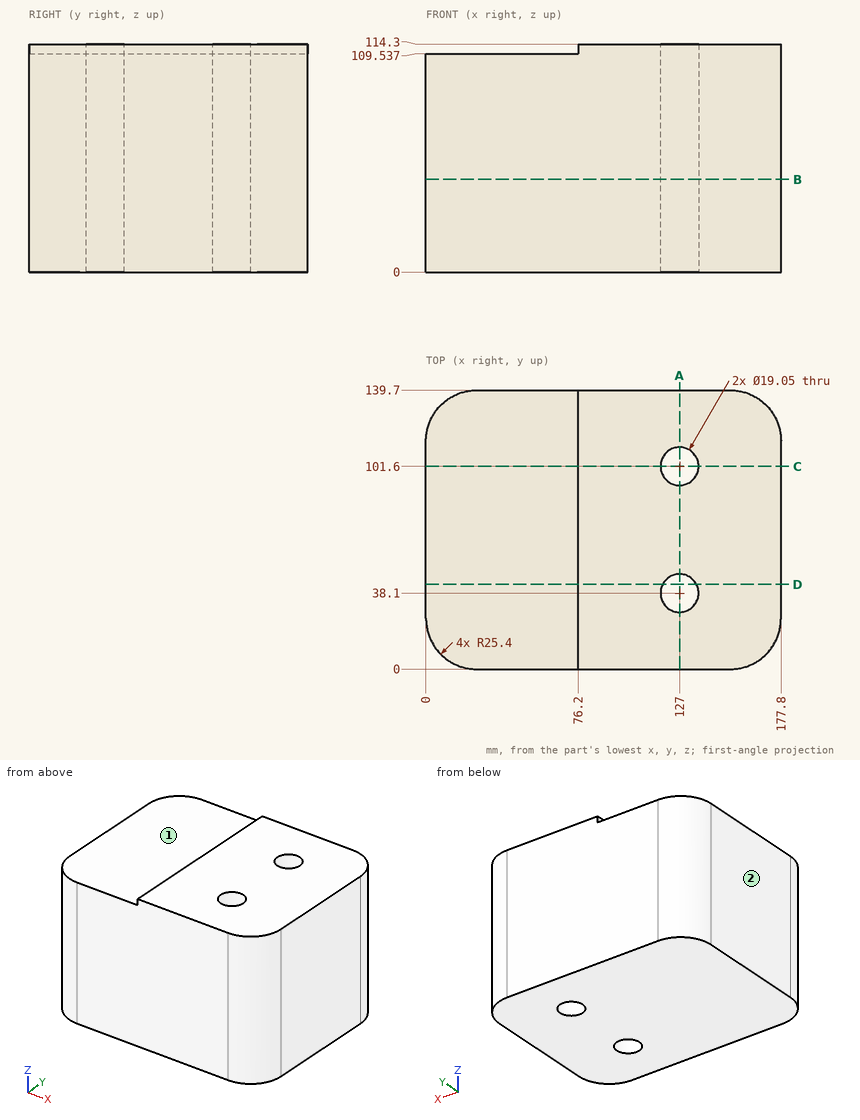
Here's the drawing with two shaded views (mm, measured from the low corner). I have some questions. A direction names the side the tool comes from. Coordinates: 2 decimals unless noted, no trailing zeros. Write each loop counter-clockwise with the first axis right and the second up, starting at its lowest first coordinate (ties: lowest second). Pieces come first, ordered by that corner, then holes.
Item 1: I want a section at C-C on y = 101.6. Write out the boundary of the cut face in (x, z) (1 decimal), and give its area (3 significant figures).
Item 2: Will these pins go through, and if not, where does the flat tip stop? pin 1 (23 mm diameter, centred on x = 25, y = 65.5, fed in from +Z); pin 2 (1 mm diameter, centred on y = 123, z = 100, fed in from -X); pin 3 (2.5 mm diameter, centred on y = 68.5, z = 111.5, fed in from -X).
Item 3: I want a section at A-A on x = 127. Write out the boundary of the cut face in (y, z) (1 decimal).
Item 4: On a 3-axis mill with a long thin cutter (end or side, diameter ignored), from which of +Z, -Z, +X, -X, +Y, -Y can I reach the whole of each face in a straight line? I mean the marked faces 1 and 2. Say none if no direction works.
Item 5: I want a section at B-B on z = 46.5. Count the separate pieces of the cut face and the enclosed holes in it, and give its area (3 significant figures).
Item 6: I want a section at D-D on y = 42.5. Write out the boundary of the cut face in (x, z).
Item 7: If I drill on line 1 (Y direction, x = 127, z = 52) (1 decimal); line 2 (X direction, y = 101, z = 32) (1 decimal); line 3 (Y direction, x = 122, z = 86) (1 decimal), over which ranges is the centre line in solid material (lowest first)?
Findings below:
1. outline: (0, 0) - (117.5, 0) - (117.5, 114.3) - (76.2, 114.3) - (76.2, 109.5) - (0, 109.5) - close; (136.5, 0) - (177.8, 0) - (177.8, 114.3) - (136.5, 114.3) - close
1. area: 17,800 mm2
2. pin 1: stops at z = 109.54
2. pin 2: stops at x = 1.36
2. pin 3: stops at x = 76.2
3. outline: (0, 0) - (28.6, 0) - (28.6, 114.3) - (0, 114.3) - close; (47.6, 0) - (92.1, 0) - (92.1, 114.3) - (47.6, 114.3) - close; (111.1, 0) - (139.7, 0) - (139.7, 114.3) - (111.1, 114.3) - close
4. face 1: +Z, -X, +Y, -Y
4. face 2: +Z, -Z, -X, +Y, -Y
5. separate pieces: 1
5. enclosed holes: 2
5. area: 23,700 mm2
6. outline: (0, 0) - (118.55, 0) - (118.55, 114.3) - (76.2, 114.3) - (76.2, 109.54) - (0, 109.54) - close; (135.45, 0) - (177.8, 0) - (177.8, 114.3) - (135.45, 114.3) - close
7. line 1: y = 0 to 28.6, 47.6 to 92.1, 111.1 to 139.7
7. line 2: x = 0 to 117.5, 136.5 to 177.8
7. line 3: y = 0 to 30, 46.2 to 93.5, 109.7 to 139.7
